Part model, mm, in its own coordinate system. A direction names the side the tool comes from. Round coordinates to 2 decimals unless told otherwise and drop trailing zeros. Loops run counter-clockwise (first coordinate to the right, second up) from the corner with the lowest first, then second, coordinate; pieces in that order, holes last. Notation, with made-up numbers: (-32.5, 40.25) -> (11.5, 40.25) arc R5 cw to (11.5, 45.25) -> close; hole circle Ø4 at (-28, 0.5). An arc over 180 degrees is marked (long way). Answer as CSV lines item,"result".
from build123d import *

# Parameters (mm, degrees)
BASE_DEPTH  = 160
ESQUISSE2_R = 2.5
TROU_DEPTH  = 161.225622171


with BuildPart() as part:
    # Esquisse1 → Base (new body)
    with BuildSketch(Plane(origin=(0, 0, 0), x_dir=(1, 0, 0), z_dir=(0, 1, 0))):
        Polygon((-2, -4), (-2, 3), (2, 3), (2, -4), (3.75, -4), (3.75, 4), (-3.75, 4), (-3.75, -4), align=None)
    extrude(amount=-BASE_DEPTH)

    # Esquisse2 → Trou (cut, through all)
    with BuildSketch(Plane.ZY.offset(3.75)):
        with Locations((0, -8)):
            Circle(ESQUISSE2_R)
        with Locations((0, -24)):
            Circle(ESQUISSE2_R)
        with Locations((0, -40)):
            Circle(ESQUISSE2_R)
        with Locations((0, -56)):
            Circle(ESQUISSE2_R)
        with Locations((0, -72)):
            Circle(ESQUISSE2_R)
        with Locations((0, -88)):
            Circle(ESQUISSE2_R)
        with Locations((0, -104)):
            Circle(ESQUISSE2_R)
        with Locations((0, -120)):
            Circle(ESQUISSE2_R)
        with Locations((0, -136)):
            Circle(ESQUISSE2_R)
        with Locations((0, -152)):
            Circle(ESQUISSE2_R)
    extrude(amount=-TROU_DEPTH, mode=Mode.SUBTRACT)


solid = part.part
Q1. Saw through at A-A, the plane y = -88. Write the cut outline in (x, z), then the cut area to 3 significant figures.
Geometry results:
outline,"(-3.75, -4) -> (3.75, -4) -> (3.75, -2.5) -> (2, -2.5) -> (2, -3) -> (-2, -3) -> (-2, -2.5) -> (-3.75, -2.5) -> close; (-3.75, 2.5) -> (-2, 2.5) -> (-2, 4) -> (-3.75, 4) -> close; (2, 2.5) -> (3.75, 2.5) -> (3.75, 4) -> (2, 4) -> close"
area,"14.5 mm2"
Q2. Saw through at B-B, the plane z = 0. Give the number of separate pieces and of enclosed holes in the cut face, then the cut area to 3 significant figures.
Geometry results:
separate pieces,"22"
enclosed holes,"0"
area,"385 mm2"
Q3. Which spindle directions (+Z, -Z, +X, -X, +Y, -Y) get a long thin tool onto all of the face, cutting with end or side? Do faces 1 (the face through (0, -79, -3)), 2 (the face through (-2.89, -149.52, -0.33)). Say none if no direction does.
Geometry results:
face 1,"+Z, +Y, -Y"
face 2,"+X, -X"
Q4. Saw through at D-D, the plane x = 0. Write the cut outline in (y, z).
Geometry results:
outline,"(-160, -4) -> (0, -4) -> (0, -3) -> (-160, -3) -> close"
Q5. Two-plate mould, pull along X, no slides. Class faces 3 (the face through (-3.75, -79, 0)), 4 (the face through (2.86, -58.44, -0.54)), 5 (the face through (2, -79, 0)): pulls with the +X half, pulls with the -X half, needs draft (parallel to the pull), parting line crosses it, or undercut.
Geometry results:
face 3,"pulls with the -X half"
face 4,"needs draft"
face 5,"undercut"
Q6. Drill centre lines: line 1 along X through (y, z) = (-63, -1.5); line 2 along Z through (x, y) = (2.95, -136); line 3 along Z through (x, y) = (3.5, -73). Where is each one in solid material? Low to high.
Geometry results:
line 1,"-3.75 to -2, 2 to 3.75"
line 2,"-4 to -2.5, 2.5 to 4"
line 3,"-4 to -2.29, 2.29 to 4"
Q7. Saw through at C-C, the plane y = -147. Write the cut outline in (x, z).
Geometry results:
outline,"(-3.75, -4) -> (3.75, -4) -> (3.75, 4) -> (2, 4) -> (2, -3) -> (-2, -3) -> (-2, 4) -> (-3.75, 4) -> close"
Q8. Drop a flat-ended pin along its axis: P1, Ø1, axis at x = 1, y = -57, coming from the +Z side. Give the stop position or say it passes through.
Geometry results:
P1,"z = -3"
